from build123d import *

# Parameters (mm, degrees)
BOSS_EXTRUDE1_DEPTH = 4
FILLET1_R           = 25
SKETCH3_W           = 81.141662503
SKETCH3_H           = 3.889724504
BOSS_EXTRUDE3_DEPTH = 57.201055289
SKETCH4_W           = 81.141662503
SKETCH4_H           = 5
BOSS_EXTRUDE4_DEPTH = 40
FILLET2_R           = 10
FILLET3_R           = 5


with BuildPart() as part:
    # Sketch1 → Boss-Extrude1 (new body)
    with BuildSketch(Plane.XY):
        Polygon((-71.429943593, 36.204490704), (56.570056407, 36.204490704), (59.71171891, 40.094215208), (-74.571606096, 40.094215208), align=None)
        Polygon((56.570056407, 36.204490704), (56.570056407, -40.995509296), (59.71171891, -44.8852338), (59.71171891, 40.094215208), align=None)
        Polygon((56.570056407, -40.995509296), (59.71171891, -44.8852338), (-74.571606096, -44.8852338), (-74.571606096, 40.094215208), (-71.429943593, 36.204490704), (-71.429943593, -40.995509296), align=None)
    extrude(amount=BOSS_EXTRUDE1_DEPTH)

    # Fillet1
    fillet1_edges = [part.edges().sort_by_distance(p)[0] for p in [
        (-71.429943593, 36.204490704, 2),
        (-71.429943593, -40.995509296, 2),
        (56.570056407, -40.995509296, 2),
        (56.570056407, 36.204490704, 2),
        (-74.571606096, -44.8852338, 2),
        (-74.571606096, 40.094215208, 2),
        (59.71171891, 40.094215208, 2),
        (59.71171891, -44.8852338, 2),
    ]]
    fillet(fillet1_edges, radius=FILLET1_R)

    # Sketch3 → Boss-Extrude3 (add)
    with BuildSketch(Plane(origin=(0, 0, 0), x_dir=(-1, 0, 0), z_dir=(0, 0, -1))):
        with Locations((5.859112342, 38.149352956)):
            Rectangle(SKETCH3_W, SKETCH3_H)
    extrude(amount=-BOSS_EXTRUDE3_DEPTH)

    # Sketch4 → Boss-Extrude4 (add)
    with BuildSketch(Plane(origin=(0, 36.204490704, 0), x_dir=(-1, 0, 0), z_dir=(0, -1, 0))):
        with Locations((5.859112342, -54.701055289)):
            Rectangle(SKETCH4_W, SKETCH4_H)
    extrude(amount=BOSS_EXTRUDE4_DEPTH)

    # Fillet2
    fillet2_edges = [part.edges().sort_by_distance(p)[0] for p in [
        (-46.429943593, -3.795509296, 54.701055289),
        (34.71171891, -3.795509296, 54.701055289),
    ]]
    fillet(fillet2_edges, radius=FILLET2_R)

    # Fillet3
    # the kernel refuses this fillet: 5 mm, written as the material it takes off along each edge
    with BuildSketch(Plane(origin=(34.71171891, 40.094215208, 4), x_dir=(-1, 0, 0), z_dir=(0, 0, 1)), Plane(origin=(-46.429943593, 40.094215208, 4), x_dir=(0, -1, 0), z_dir=(0, 0, 1))) as fillet3_piece_1:
        with BuildLine():
            CenterArc((FILLET3_R, FILLET3_R), FILLET3_R, 180, 90)
            Line((0, FILLET3_R), (0, 0))
            Line((0, 0), (FILLET3_R, 0))
        make_face()
    extrude(amount=65.701055289, mode=Mode.SUBTRACT)


solid = part.part
Work out the finished part from the listing and answer in its coordinate system (mm). A direction names the side the tool comes from. Give positions to 0.01 mm unless a question says otherwise; leave off trailing zeros. Order: outer loops, then holes, each group sorted by start corner. A loop starts at its lowest first (then second) coordinate and runs counter-clockwise, first axis right, second up. Notation, with made-up numbers: M 43,-29.5 L 74,-29.5 A25 cw 74,-11.5 Z; hole C 47,67 d4. An arc over 180 degrees is marked long. Return JSON: item names as keys, results as strings.
Q1. Find section B-B, the plane x = 15. Write down the section's boundary in (y, z).
Answer below:
{"outline": "M -44.89,0 L -41,0 L -41,4 L -44.89,4 Z; M -3.8,52.2 L 36.2,52.2 L 36.2,0 L 40.09,0 L 40.09,57.2 L -3.8,57.2 Z"}
Q2. Find the intervals of material crossed by line 1 along Y through (x, z) = (22, 26.5); line 2 along Z through (x, y) = (22.5, -2.5); line 3 along Y through (x, z) = (32.5, 21), in increasing order. Write a range as [from, to].
Answer below:
{"line 1": "y = [36.2, 40.09]", "line 2": "z = [52.2, 57.2]", "line 3": "y = [36.2, 39.24]"}
Q3. Each of these flat-tipped pins is pushed along its axis until it touches: pin 1 (20 mm diameter, centred on x = -4, y = 17, fed in from -Z); pin 2 (4 mm diameter, centred on x = 35, y = 17.5, fed in from +Z); pin 3 (1.5 mm diameter, centred on y = 26.5, z = 54.5, fed in from -X); pin 4 (2.5 mm diameter, centred on x = 1.5, z = 54.5, fed in from -Y). Where does it stop, or does it pass through?
Answer below:
{"pin 1": "stops at z = 52.2", "pin 2": "stops at z = 57.2", "pin 3": "stops at x = -46.43", "pin 4": "stops at y = -3.8"}
Q4. Which of the six approach directions +Z, -Z, +X, -X, +Y, -Y give full straight-line access (tool end or side, diameter ignored) to faces 4 (the face through (52.58, -37.37, 2.03)), 5 (the face through (-63.91, 29.08, 2.03))?
Answer below:
{"face 4": "+Z, -Z, +X, -Y", "face 5": "+Z, -Z"}
Q5. Find section D-D, the plane x = -58.5. Write down the section's boundary in (y, z), and give its area (3 significant figures).
Answer below:
{"outline": "M -43.24,0 L -37.89,0 L -37.89,4 L -43.24,4 Z; M 33.1,0 L 38.45,0 L 38.45,4 L 33.1,4 Z", "area": "42.8 mm^2"}
Q6. Find section C-C, the plane y = 23. Write down the section's boundary in (x, z).
Answer below:
{"outline": "M -73.29,0 L -68.47,0 L -68.47,4 L -73.29,4 Z; M -46.43,52.2 L 34.71,52.2 L 34.71,57.2 L -46.43,57.2 Z; M 53.61,0 L 58.43,0 L 58.43,4 L 53.61,4 Z"}
Q7. Find section A-A, the plane y = -12. Write down the section's boundary in (x, z).
Answer below:
{"outline": "M -74.57,0 L -71.43,0 L -71.43,4 L -74.57,4 Z; M 56.57,0 L 59.71,0 L 59.71,4 L 56.57,4 Z"}
Q8. The mould has two halves that part along X. Classify faces 1 (the face through (-44.926, 38.668, 30.228)), 2 (the face through (33.286, 38.591, 30.228)), 3 (the face through (49.44, -33.48, 2.03)): pulls with the +X half, pulls with the -X half, needs draft (parallel to the pull), parting line crosses it, or undercut.
Answer below:
{"face 1": "pulls with the -X half", "face 2": "pulls with the +X half", "face 3": "undercut"}
